```python
from build123d import *

# Parameters (mm, degrees)
SKETCH4_W           = 150
SKETCH4_H           = 150
BOSS_EXTRUDE1_DEPTH = 30
SHELL2_T            = -5
SKETCH5_R           = 11
CUT_EXTRUDE1_DEPTH  = 10
SKETCH6_W           = 70
SKETCH6_H           = 24
CUT_EXTRUDE2_DEPTH  = 10
SKETCH7_R           = 6
CUT_EXTRUDE3_DEPTH  = 10
SKETCH8_R           = 2.5
CUT_EXTRUDE4_DEPTH  = 10
SKETCH10_R          = 2
CUT_EXTRUDE5_DEPTH  = 10


with BuildPart() as part:
    # Sketch4 → Boss-Extrude1 (new body)
    with BuildSketch(Plane.XY):
        Rectangle(SKETCH4_W, SKETCH4_H)
    extrude(amount=BOSS_EXTRUDE1_DEPTH)

    # Shell2
    shell2_openings = [part.faces().sort_by_distance(p)[0] for p in [
        (0, 0, 30),
    ]]
    offset(amount=SHELL2_T, openings=shell2_openings, kind=Kind.INTERSECTION)

    # Sketch5 → Cut-Extrude1 (cut)
    with BuildSketch(Plane(origin=(0, 0, 0), x_dir=(-1, 0, 0), z_dir=(0, 0, -1))):
        with Locations((0, 55.503756803)):
            Circle(SKETCH5_R)
    extrude(amount=-CUT_EXTRUDE1_DEPTH, mode=Mode.SUBTRACT)

    # Sketch6 → Cut-Extrude2 (cut)
    with BuildSketch(Plane(origin=(0, 0, 0), x_dir=(-1, 0, 0), z_dir=(0, 0, -1))):
        with Locations((0, 6.168751782)):
            Rectangle(SKETCH6_W, SKETCH6_H)
    extrude(amount=-CUT_EXTRUDE2_DEPTH, mode=Mode.SUBTRACT)

    # Sketch7 → Cut-Extrude3 (cut)
    with BuildSketch(Plane(origin=(0, 0, 0), x_dir=(-1, 0, 0), z_dir=(0, 0, -1))):
        with Locations((52.142360775, 21.195860283)):
            Circle(SKETCH7_R)
    extrude(amount=-CUT_EXTRUDE3_DEPTH, mode=Mode.SUBTRACT)

    # Sketch8 → Cut-Extrude4 (cut)
    with BuildSketch(Plane(origin=(0, 0, 0), x_dir=(-1, 0, 0), z_dir=(0, 0, -1))):
        with Locations((-48.952452987, -41.390507081)):
            Circle(SKETCH8_R)
    extrude(amount=-CUT_EXTRUDE4_DEPTH, mode=Mode.SUBTRACT)

    # Sketch10 → Cut-Extrude5 (cut)
    with BuildSketch(Plane(origin=(0, 0, 0), x_dir=(-1, 0, 0), z_dir=(0, 0, -1))):
        with Locations((55.147282701, -52.031429677)):
            Circle(SKETCH10_R)
        with Locations((55.147282701, -38.731179224)):
            Circle(SKETCH10_R)
    extrude(amount=-CUT_EXTRUDE5_DEPTH, mode=Mode.SUBTRACT)


solid = part.part
```
For this review, take the finished solid that the model builds, in its own axes (mm). A direction names the side the tool comes from. Round coordinates to 2 decimals unless told otherwise and drop trailing zeros. Write each loop counter-clockwise with the first axis right and the second up, starting at its lowest first coordinate (ties: lowest second). Pieces come first, ordered by that corner, then holes.
1) Insertion check: pin 1 Ø8 at (x, y) = (-54, -5) entering from +Z; pin 2 Ø1.5 at (x, y) = (34.5, -6.5) entering from -Z. Each pin has a flat end and moves straight along its axis. Give the tip position at first contact, or say it passes through.
Answer below:
pin 1: stops at z = 5
pin 2: stops at z = 0
2) For line 1 along Y through (x, z) = (0, 2.3); line 2 along Y through (x, z) = (-60, 14), list the stretches that pass through material, from the lowest coordinate up.
Answer below:
line 1: y = -75 to -5.83, 18.17 to 44.5, 66.5 to 75
line 2: y = -75 to -70, 70 to 75
3) Take a section at D-D on x = -60.5. Give the boundary of the cut face in (y, z), then the cut area to 3 significant figures.
Answer below:
outline: (-75, 0) - (75, 0) - (75, 30) - (70, 30) - (70, 5) - (-70, 5) - (-70, 30) - (-75, 30) - close
area: 1,000 mm2
4) Take a section at A-A on x = 0. Give the boundary of the cut face in (y, z).
Answer below:
outline: (-75, 0) - (-5.83, 0) - (-5.83, 5) - (-70, 5) - (-70, 30) - (-75, 30) - close; (18.17, 0) - (44.5, 0) - (44.5, 5) - (18.17, 5) - close; (66.5, 0) - (75, 0) - (75, 30) - (70, 30) - (70, 5) - (66.5, 5) - close
5) Take a section at B-B on z = 12.5. Give the boundary of the cut face in (x, y), then the cut area to 3 significant figures.
Answer below:
outline: (-75, -75) - (75, -75) - (75, 75) - (-75, 75) - close; hole (-70, -70) - (70, -70) - (70, 70) - (-70, 70) - close
area: 2,900 mm2
6) Mouldability with a two-part tool opening along Y and no side actions: class faces 4 (the face through (-1, -75, 15)), 5 (the face through (-1, 75, 15)), 6 (the face through (-75, -1, 15)), 7 (the face through (-57.055, -38.13, 2.465)) as +Y half, -Y half, draft (parallel to the pull), parting line (faces both ways), or undercut.
Answer below:
face 4: -Y half
face 5: +Y half
face 6: draft
face 7: undercut
7) Machinability: for faces 1 (the face through (-1, -15, 5)), 2 (the face through (-1, -16, 0)), 3 (the face through (0, -5.831, 2)), which of the approach directions +Z, -Z, +X, -X, +Y, -Y give a long, thin tool a straight path to every point of the face, cutting with its end or side? Answer none if there is none.
Answer below:
face 1: +Z
face 2: -Z, +X, -X, +Y, -Y
face 3: +Z, -Z
8) Take a section at C-C on x = -15. Give the boundary of the cut face in (y, z).
Answer below:
outline: (-75, 0) - (-5.83, 0) - (-5.83, 5) - (-70, 5) - (-70, 30) - (-75, 30) - close; (18.17, 0) - (75, 0) - (75, 30) - (70, 30) - (70, 5) - (18.17, 5) - close
